Can you work these out from the model? Positions are in its coordinate system, mm. A direction names the side the tool comes from. Give positions to 0.01 mm unless a question says otherwise; leave off trailing zeros. Order: outer loops, then holes, each group sorted by start corner. A loop starts at its lowest first (then second) coordinate and runs counter-clockwise, first axis right, second up. Notation, with made-up numbers: M 30.5,20.5 L 65.5,20.5 A18 ccw 65.5,48.5 Z; hole C 88,59 d2. An arc over 180 degrees is marked long. Use one line per item in the form item = value. Start each with the question number.
1. For faces 1 (the face through (10, 0.3, -19.5)), 2 (the face through (7, 0, -19)), which set-ups out of +Z, -Z, +X, -X, +Y, -Y let a thin tool reach every point of the face, with its end or its side?
2. Will these pins go through, and if not, where does the flat tip stop? P1, Ø0.5, axis at x = 5.5, z = 13.5, coming from the -Y side; P2, Ø1.1, axis at x = 5, z = 19.5, coming from the +Y side.
3. I need wall thicknesses on L1, parallel to Y at x = 0.8, z = 15.5; L2, parallel to Z at x = 1.1, y = -16; L3, parallel to Z at x = 2.75, y = 0. Which ranges of each line are inside material? Lowest first, please.
4. I want a section at D-D, the plane z = -12.5. List the corners of the cut face in (x, y) for me, and give its area (3 significant figures).
5. I want a section at B-B, the plane z = 0. List the corners of the cut face in (x, y) for me, and give its area (3 significant figures).
6. I want a section at C-C, the plane x = 7.25. Count the separate pieces of the cut face and the enclosed holes in it, and give its area (3 significant figures).
7. We'd pull the mould along Z, two halves only. Please class faces 3 (the face through (10, -13.4, -1.5)), 4 (the face through (1.521, -17.983, 15.24)): +Z half, -Z half, draft (parallel to the pull), parting line (faces both ways), or undercut.
8. I want a section at A-A, the plane z = 15.5. List the corners of the cut face in (x, y) for me, and give its area (3 significant figures).
Autodesk Inventor part; units mm, degrees
ref_plane "YZ Plane" through (0, 0, 0) normal (1, 0, 0) x (0, 1, 0)
ref_plane "XZ Plane" through (0, 0, 0) normal (0, 1, 0) x (-1, 0, 0)
ref_plane "XY Plane" through (0, 0, 0) normal (0, 0, 1) x (1, 0, 0)
sketch "Szkic1" plane through (0, 0, 0) normal (1, 0, 0) x (0, 1, 0)
  line L0 (20, 20) -> (-20, 20)
  line L1 (-20, 20) -> (-20, -20)
  line L2 (-20, -20) -> (20, -20)
  line L3 (20, -20) -> (20, 20)
  line L4 (20, 0) -> (0, 0) construction
  line L5 (0, 0) -> (0, -20) construction
  dimension "d0" = 40
  dimension "d1" = 40
extrude "Wyciągnięcie proste1" add sketch "Szkic1" along normal blind 2
sketch "Szkic4" plane through (0, 20, 20) normal (0, 1, 0) x (1, 0, 0)
  line L0 (0, 40) -> (2, 40)
  line L1 (2, 40) -> (10, 40)
  line L2 (10, 40) -> (10, 39)
  line L3 (10, 39) -> (3, 39)
  line L4 (3, 39) -> (3, 37)
  line L5 (3, 37) -> (2, 37)
  line L6 (2, 40) -> (2, 37)
  line L7 (2, 0) -> (2, 40)
  point P0 (0, 20)
  dimension "d27" = 8
  dimension "d29" = 2
  dimension "d30" = 1
  dimension "d31" = 1
extrude "Wyciągnięcie proste2" add sketch "Szkic4" against normal up to surface (40 mm away)
pattern_linear "Szyk prostokątny1" count 13 spacing 3 along (0, 0, 1) of "Wyciągnięcie proste2"
sketch "Szkic5" plane through (0, 20, 20) normal (0, 1, 0) x (1, 0, 0)
  line L0 (2, 1) -> (2, 0)
  line L1 (2, 1) -> (10, 1)
  line L2 (10, 1) -> (10, 0)
  line L3 (10, 0) -> (2, 0)
  line L4 (2, 0) -> (2, 1)
  line L5 (10, 3) -> (10, 4)
  line L6 (0, 0) -> (2, 0)
  point P0 (0, 20)
  point P1 (1, 0)
extrude "Wyciągnięcie proste3" add sketch "Szkic5" against normal up to surface (40 mm away)
sketch "Szkic6" plane through (0, 0, 0) normal (-1, 0, 0) x (0, 0, 1)
  point P0 (0, 0)
  point P1 (0, 0)
hole "Otwór1" at (0, 0, 0) direction (1, 0, 0) diameter 14.5 end through all
sketch "Szkic7" plane through (0, 0, 0) normal (-1, 0, 0) x (0, 0, 1)
  line L0 (0, 0) -> (-20, 0) construction
  line L1 (-20, -20) -> (-20, 20)
  line L2 (20, 20) -> (20, -20)
  point P0 (15.5, -16)
  point P1 (15.5, 16)
  dimension "d46" = 32
  dimension "d47" = 4.5
hole "Otwór2" at (0, -16, 15.5) at (0, 16, 15.5) direction (1, 0, 0) diameter 4 end through all
sketch "Szkic8" plane through (10, 20, 20) normal (1, 0, 0) x (0, 0, -1)
  line L0 (0, 0) -> (0, -40)
  line L1 (7, 0) -> (0, 0)
  line L2 (0, 0) -> (0, -9)
  line L3 (0, -9) -> (7, -9)
  line L4 (7, -9) -> (7, 0)
  line L5 (7, 0) -> (7, -40)
  line L6 (0, -40) -> (7, -40)
  line L7 (7, -40) -> (7, -31)
  line L8 (7, -31) -> (0, -31)
  line L9 (0, -31) -> (0, -40)
  point P0 (20, -20)
  dimension "d56" = 9
  dimension "d57" = 9
extrude "Wyciągnięcie proste4" cut sketch "Szkic8" against normal up to surface (7 mm away) contours L1 L4 L3 L0 | L8 L5 L6 L0
properties part number "36_radiator"
Check result:
q1.face_1 = +Z, -Z, +X, +Y, -Y
q1.face_2 = +X, +Y, -Y
q2.P1 = -11
q2.P2 = 11
q3.L1 = -20 to -18, -14 to 14, 18 to 20
q3.L2 = -20 to 13.5, 17.5 to 20
q3.L3 = -20 to -7.25, 7.25 to 20
q4.outline = M 0,-20 L 3,-20 L 3,20 L 0,20 Z
q4.area = 120 mm2
q5.outline = M 0,-20 L 3,-20 L 3,-7.25 L 0,-7.25 Z; M 0,7.25 L 3,7.25 L 3,20 L 0,20 Z
q5.area = 76.5 mm2
q6.separate_pieces = 18
q6.enclosed_holes = 0
q6.area = 454 mm2
q7.face_3 = draft
q7.face_4 = undercut
q8.outline = M 0,-20 L 3,-20 L 3,-18 L 0,-18 Z; M 0,-14 L 3,-14 L 3,14 L 0,14 Z; M 0,18 L 3,18 L 3,20 L 0,20 Z
q8.area = 96.0 mm2
